```python
from build123d import *

# Parameters (mm, degrees)
F0_R            = 6.5
F1_DEPTH        = 7
F5_DEPTH        = 7.001
F5_COPIES_COUNT = 12


# Not quite as in the source:
# - a pattern or mirror of a feature is missing from the dataset's text; its kind, count and spacing are read off the source's solid


with BuildPart() as f1:
    # F0 (on Front) → F1 (new body)
    with BuildSketch(Plane.XZ):
        Circle(F0_R)
        Polygon((-1.75, 0.5), (-0.5, 0.5), (-0.5, 1.75), (0.5, 1.75), (0.5, 0.5), (1.75, 0.5), (1.75, -0.5), (0.5, -0.5), (0.5, -1.75), (-0.5, -1.75), (-0.5, -0.5), (-1.75, -0.5), align=None, mode=Mode.SUBTRACT)
    extrude(amount=F1_DEPTH)

    # F2 (on Right) → F3 (revolve, cut)
    with BuildSketch(Plane.YZ):
        Polygon((-7, 8), (-7, 5), (-6.375, 6.0825317547), (-4.875, 6.0825317547), (-4.875, 6.5), (-2.125, 6.5), (-2.125, 6.0825317547), (-0.625, 6.0825317547), (0, 5), (0, 8), align=None)
    revolve(axis=Axis((0, 2.603987056, 0), (0, 1, 0)), mode=Mode.SUBTRACT)

    # F4 (on Front) → F5 (cut, through all)
    with BuildSketch(Plane.XZ):
        with BuildLine():
            Line((0.5, 3.9686269666), (1, 6.4226162893))
            ThreePointArc((1, 6.4226162893), (0, 6.5), (-1, 6.4226162893))
            Line((-1, 6.4226162893), (-0.5, 3.9686269666))
            ThreePointArc((-0.5, 3.9686269666), (0, 4), (0.5, 3.9686269666))
        make_face()
    f5 = extrude(amount=F5_DEPTH, mode=Mode.SUBTRACT)

    # F5_copies: F5 ×12 about axis
    f5_copies_axis = Axis((0, 0, 0), (0, 1, 0))
    for i in range(1, F5_COPIES_COUNT):
        add(f5.rotate(f5_copies_axis, i * 360 / F5_COPIES_COUNT), mode=Mode.SUBTRACT)


solid = f1.part
```
Geometry: final body of the model. Coordinates: model frame, mm. A direction names the side the tool comes from. Coordinates: 2 decimals unless noted, no trailing zeros. Loops run counter-clockwise (first coordinate to the right, second up) from the corner with the lowest first, then second, coordinate; pieces in that order, holes last. Notation, with made-up numbers: (14.5, 63) -> (60.5, 63) arc R27 cw to (60.5, 80) -> close; hole circle Ø3 at (68, -3). An arc over 180 degrees is marked (long way). Use a Markdown table: item, result. Add a question column.
(1) Pin query (flat end, axial travel): pin 1 Ø0.6 at (x, z) = (-6, 2) entering from +Y; pin 2 Ø1 at (y, z) = (-3.5, 1.5) entering from -X; pin 3 Ø1 at (x, z) = (4.5, -4) entering from +Y; pin 4 Ø0.8 at (y, z) = (-5, 0) entering from +X. Return the tip coordinate at first contact, or that it passes through.
(2) Mould query, pull axis Z, two halves, no side actions, for faces 6 (the conical face through (-3.91, -0.31, -3.92)), 7 (the cylindrical face through (-5.878, -1.364, 1.565)), 8 (the flat face through (-4.4, -4.875, -4.5)), 9 (the flat face through (-1.866, -3.451, -4.627)). Classes: pulls with the +Z half, pulls with the -Z half, needs draft (parallel to the pull), parting line crosses it, or undercut.
(3) Access query for faces 1 (the flat face through (0.698, -3.451, -4.94)), 2 (the flat face through (-4.94, -3.451, -0.698)), 3 (the flat face through (-0.5, -3, 1)), 4 (the cylindrical face through (-4.3, -5.6, 4.3)), 5 (the cylindrical face through (4.3, -1.4, 4.3)). Directions: +Z, -Z, +X, -X, +Y, -Y. A direction counts if a zero-diameter tool reaches every point of the face in a straight line with its end or side. Return the directions, or none.
(4) Line query: line 1 along Z through (x, y) = (3.5, -2.75); line 2 along Z through (x, y) = (4.25, -2.5); line 3 along X through (y, z) = (-4.25, 0). Output: solid intervals per line, ascending.
(5) Section query A-A, the plane z = 2.75. Return loops of the section in (x, y).
Answer:
| question | item | result |
|---|---|---|
| 1 | pin 1 | stops at y = -0.59 |
| 1 | pin 2 | stops at x = -6.42 |
| 1 | pin 3 | stops at y = -0.3 |
| 1 | pin 4 | stops at x = 4 |
| 2 | face 6 | pulls with the -Z half |
| 2 | face 7 | pulls with the +Z half |
| 2 | face 8 | needs draft |
| 2 | face 9 | undercut |
| 3 | face 1 | -Z, +Y, -Y |
| 3 | face 2 | -X, +Y, -Y |
| 3 | face 3 | +Y, -Y |
| 3 | face 4 | +Z, -X, -Y |
| 3 | face 5 | +Z, +X, +Y |
| 4 | line 1 | z = -4.41 to -2.69, -1.94 to 1.94, 2.69 to 4.41 |
| 4 | line 2 | z = -4.92 to -3.36, -1.74 to -0.56, 0.56 to 1.74, 3.36 to 4.92 |
| 4 | line 3 | x = -4 to -1.75, 1.75 to 4 |
| 5 | outline | (-3.56, -7) -> (3.56, -7) -> (3.56, 0) -> (-3.56, 0) -> close |
